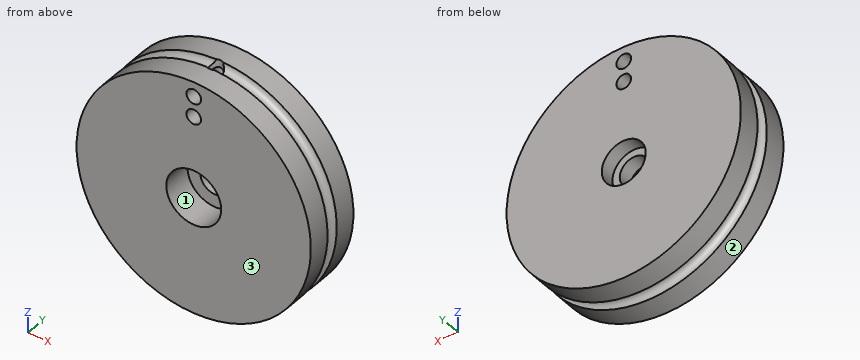
from build123d import *

# Parameters (mm, degrees)
SKETCH1_R           = 10.16
SKETCH1_R_2         = 2.38125
BOSS_EXTRUDE1_DEPTH = 5.08
BOSS_EXTRUDE2_START = -2.54
SKETCH2_R           = 2.38125
SKETCH2_R_2         = 1.27
BOSS_EXTRUDE2_DEPTH = 2.54
SKETCH3_R           = 1.905
CUT_EXTRUDE1_DEPTH  = 1.27
SKETCH4_R           = 0.552075519
SKETCH5_R           = 0.635
CUT_EXTRUDE2_DEPTH  = 16.24
SKETCH6_R           = 0.635
CUT_EXTRUDE3_DEPTH  = 3.683


with BuildPart() as part:
    # Sketch1 → Boss-Extrude1 (new body)
    with BuildSketch(Plane(origin=(0, 0, 0), x_dir=(1, 0, 0), z_dir=(0, 1, 0))):
        with Locations(Location((0, 0, 0), (0, 0, 270))):
            Circle(SKETCH1_R)
        with Locations(Location((0, 0, 0), (0, 0, 270))):
            Circle(SKETCH1_R_2, mode=Mode.SUBTRACT)
    extrude(amount=BOSS_EXTRUDE1_DEPTH)

    # Sketch2 → Boss-Extrude2 (add)
    with BuildSketch(Plane(origin=(0, 5.08, 0), x_dir=(1, 0, 0), z_dir=(0, 1, 0)).offset(BOSS_EXTRUDE2_START)):
        with Locations(Location((0, 0, 0), (0, 0, 270))):
            Circle(SKETCH2_R)
        with Locations(Location((0, 0, 0), (0, 0, 270))):
            Circle(SKETCH2_R_2, mode=Mode.SUBTRACT)
    extrude(amount=BOSS_EXTRUDE2_DEPTH)

    # Sketch3 → Cut-Extrude1 (cut)
    with BuildSketch(Plane(origin=(0, 5.08, 0), x_dir=(1, 0, 0), z_dir=(0, 1, 0))):
        with Locations(Location((0, 0, 0), (0, 0, 270))):
            Circle(SKETCH3_R)
    extrude(amount=-CUT_EXTRUDE1_DEPTH, mode=Mode.SUBTRACT)

    # Sketch4 → Cut-Revolve1 (revolve, cut)
    with BuildSketch(Plane.XY, mode=Mode.PRIVATE) as cut_revolve1_sk:
        with Locations((10.16, 2.54)):
            Circle(SKETCH4_R)
    revolve(cut_revolve1_sk.sketch.rotate(Axis((0, 6.474479785, 0), (0, -1, 0)), 90), axis=Axis((0, 6.474479785, 0), (0, -1, 0)), mode=Mode.SUBTRACT)

    # Sketch5 → Cut-Extrude2 (cut, through all)
    with BuildSketch(Plane(origin=(0, 5.08, 0), x_dir=(1, 0, 0), z_dir=(0, 1, 0))):
        with Locations(Location((0, -8.89, 0), (0, 0, 270))):
            Circle(SKETCH5_R)
        with Locations(Location((0, -7.112, 0), (0, 0, 270))):
            Circle(SKETCH5_R)
    extrude(amount=-CUT_EXTRUDE2_DEPTH, mode=Mode.SUBTRACT)

    # Sketch6 → Cut-Extrude3 (cut)
    with BuildSketch(Plane.XY.offset(10.16)):
        with Locations((0, 2.54)):
            Circle(SKETCH6_R)
    extrude(amount=-CUT_EXTRUDE3_DEPTH, mode=Mode.SUBTRACT)


solid = part.part
Source: CAD feature listing. Evaluate the final solid. Frame: model axes, mm. Face numbers are marked on the shaded views. Give positions to 0.01 mm unless a question says otherwise; leave off trailing zeros. Write each loop counter-clockwise with the first axis right and the second up, starting at its lowest first coordinate (ties: lowest second). Pieces come first, ordered by that corner, then holes. Notation, with made-up numbers: M 39.5,11.25 L 55.5,11.25 A28 ccw 55.5,45.25 Z; hole C 61,63.25 d8. An arc over 180 degrees is marked long. Answer as a JSON object with one key per item and string values.
Q1. Contact query for flat-ended pins moving along their axis: P1, Ø1, axis at x = 0, y = 2.54, coming from the +Z side; P2, Ø2, axis at x = -4.5, y = 2.5, coming from the -Z side; P3, Ø2, axis at y = 3.5, z = -4, coming from the -X side. Output: stop coordinate, or through.
Geometry check:
{"P1": "stops at z = 6.48", "P2": "stops at z = -9.49", "P3": "stops at x = -9.71"}
Q2. Cut plane C-C, the plane y = 4.3. Return the cut outline in (x, z) (3 decimals), then the cut area to 3 significant figures.
Geometry check:
{"outline": "C 0,0 d20.32; hole C 0,0 d3.81; hole C 0,7.112 d1.27; hole C 0,8.89 d1.27", "area": "310 mm^2"}
Q3. Cut plane A-A, the plane z = 0. Return the cut outline in (x, y) (3 decimals), then the cut area to 3 significant figures.
Geometry check:
{"outline": "M -10.16,0 L -2.381,0 L -2.381,2.54 L -1.27,2.54 L -1.27,3.81 L -1.905,3.81 L -1.905,5.08 L -10.16,5.08 L -10.16,3.092 A0.552 cw -10.16,1.988 Z; M 1.27,2.54 L 2.381,2.54 L 2.381,0 L 10.16,0 L 10.16,1.988 A0.552 cw 10.16,3.092 L 10.16,5.08 L 1.905,5.08 L 1.905,3.81 L 1.27,3.81 Z", "area": "82.1 mm^2"}
Q4. Cut plane B-B, the plane y = 2.8. Return the cut outline in (x, z) (3 decimals).
Geometry check:
{"outline": "M -0.579,6.477 L -0.579,6.852 A0.635 cw -0.579,7.372 L -0.579,8.63 A0.635 cw -0.579,9.15 L -0.579,9.656 A9.673 ccw long 0.579,9.656 L 0.579,9.15 A0.635 cw 0.579,8.63 L 0.579,7.372 A0.635 cw 0.579,6.852 L 0.579,6.477 Z; hole C 0,0 d2.54"}
Q5. Mould query, pull axis X, two halves, no side actions, for the marked faces 1, 2 and 3. Classes: +X half, -X half, draft (parallel to the pull), parting line (faces both ways), or undercut.
Geometry check:
{"face 1": "undercut", "face 2": "parting line", "face 3": "draft"}
Q6. Ray query, line 1 along Z through (x, y) = (0.5, 2.6); line 2 along X through (y, z) = (0.9, 8.89) (3 decimals); line 3 along Y through (x, z) = (5.75, 8.25). Return the intervals inside material, ascending.
Geometry check:
{"line 1": "z = -9.6 to -1.17, 1.17 to 6.48", "line 2": "x = -4.919 to -0.635, 0.635 to 4.919", "line 3": "y = 0 to 2, 3.08 to 5.08"}
